```python
from build123d import *

# Parameters (mm, degrees)
BOSS_EXTRUDE1_DEPTH = 5
SKETCH1_13_R        = 1.1
CUT_EXTRUDE2_DEPTH  = 10
FILLET1_R           = 2
BOSS_EXTRUDE2_DEPTH = 14
SKETCH2_R           = 1.35
CUT_EXTRUDE3_DEPTH  = 110
FILLET2_R           = 5
CUT_EXTRUDE4_START  = 200
SKETCH2_3_R         = 2.75
CUT_EXTRUDE4_DEPTH  = 111


with BuildPart() as part:
    # Sketch1 → Boss-Extrude1 (new body)
    with BuildSketch(Plane.XY):
        with BuildLine():
            Line((27.361611466, 75.175409663), (32.833933759, 90.210491595))
            ThreePointArc((32.833933759, 90.210491595), (9.201192242, 95.558035043), (-15.017708644, 94.818080697))
            Line((-15.017708644, 94.818080697), (-12.514757203, 79.015067248))
            ThreePointArc((-12.514757203, 79.015067248), (7.667660202, 79.631695869), (27.361611466, 75.175409663))
        make_face()
    extrude(amount=BOSS_EXTRUDE1_DEPTH)

    # Sketch1<13> → Cut-Extrude2 (cut)
    with BuildSketch(Plane.XY):
        with BuildLine():
            ThreePointArc((13.453363993, 84.941197291), (19.959187303, 83.651843029), (26.346302102, 81.864964213))
            Line((26.346302102, 81.864964213), (27.571711502, 85.672636967))
            ThreePointArc((27.571711502, 85.672636967), (20.887521597, 87.542626426), (14.079101854, 88.891950654))
            Line((14.079101854, 88.891950654), (13.453363993, 84.941197291))
        make_face()
        with Locations((8, 88)):
            Circle(SKETCH1_13_R)
    extrude(amount=CUT_EXTRUDE2_DEPTH, mode=Mode.SUBTRACT)

    # Fillet1
    fillet1_edges = [part.edges().sort_by_distance(p)[0] for p in [
        (26.346302102, 81.864964213, 2.5),
        (27.571711502, 85.672636967, 2.5),
        (14.079101854, 88.891950654, 2.5),
        (13.453363993, 84.941197291, 2.5),
    ]]
    fillet(fillet1_edges, radius=FILLET1_R - 0.0001)  # a hair under: the kernel refuses the full size

    # Sketch1<14> → Boss-Extrude2 (add)
    with BuildSketch(Plane.XY):
        with BuildLine():
            ThreePointArc((-0.5, 93.344488005), (-9.226985142, 88), (-0.5, 82.655511995))
            Line((-0.5, 82.655511995), (-0.5, 93.344488005))
        make_face()
        with BuildLine():
            Line((-0.5, 93.344488005), (-0.5, 82.655511995))
            ThreePointArc((-0.5, 82.655511995), (1.889747744, 84.866464525), (2.773014858, 88))
            ThreePointArc((2.773014858, 88), (1.889747744, 91.133535475), (-0.5, 93.344488005))
        make_face()
    extrude(amount=BOSS_EXTRUDE2_DEPTH)

    # Sketch2 → Cut-Extrude3 (cut)
    with BuildSketch(Plane(origin=(0, 0, 0), x_dir=(1, 0, 0), z_dir=(0, 1, 0))):
        with Locations(Location((-3.226985142, -8, 0), (0, 0, 90))):
            Circle(SKETCH2_R)
    extrude(amount=CUT_EXTRUDE3_DEPTH, mode=Mode.SUBTRACT)

    # Fillet2
    fillet2_edges = [part.edges().sort_by_distance(p)[0] for p in [
        (27.361611466, 75.175409663, 2.5),
        (-12.514757203, 79.015067248, 2.5),
        (-15.017708644, 94.818080697, 2.5),
        (32.833933759, 90.210491595, 2.5),
    ]]
    fillet(fillet2_edges, radius=FILLET2_R)

    # Sketch2<3> → Cut-Extrude4 (cut)
    with BuildSketch(Plane(origin=(0, 0, 0), x_dir=(1, 0, 0), z_dir=(0, 1, 0)).offset(CUT_EXTRUDE4_START)):
        with Locations(Location((-3.226985142, -8, 0), (0, 0, 270))):
            Circle(SKETCH2_3_R)
    extrude(amount=-CUT_EXTRUDE4_DEPTH, mode=Mode.SUBTRACT)


solid = part.part
```
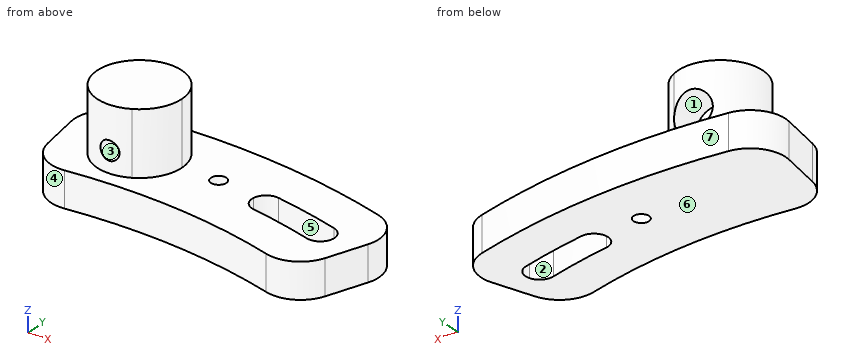
Work out the finished part from the listing and answer in its coordinate system (mm). Face numbers are marked on the shaded views. A direction names the side the tool comes from. Coordinates: 2 decimals unless noted, no trailing zeros. Order: outer loops, then holes, each group sorted by start corner. A loop starts at its lowest first (then second) coordinate and runs counter-clockwise, first axis right, second up. Notation, with made-up numbers: (79, 1.25) - (125, 1.25) arc R8 cw to (125, 6.25) - close; hole circle Ø3 at (-28, 40). An arc over 180 degrees is marked (long way). Answer as a JSON object with one key per item and string values.
1. Find section A-A on z = 1.5. Count the separate pieces of the cut face and the enclosed holes in it, plus the area to 3 significant figures.
Output values:
{"separate pieces": "1", "enclosed holes": "2", "area": "637 mm²"}
2. Find section C-C on y = 91. Determine the outline of the cut face in (x, z).
Output values:
{"outline": "(-14.25, 0) - (29.5, 0) - (29.5, 5) - (1.97, 5) - (1.97, 14) - (-8.42, 14) - (-8.42, 5) - (-14.25, 5) - close; hole circle Ø5.5 at (-3.23, 8)"}
3. Find section D-D on z = 11.25. Determine the outline of the cut face in (x, y).
Output values:
{"outline": "circle Ø12 at (-3.23, 88)"}
4. A tool of negligible diameter and unlimited length cuts with its end or side. For the marked faces 1, 2 and 3, from which of +Z, -Z, +X, -X, +Y, -Y can it reach the whole face along a straight path? Write none if from no direction.
Output values:
{"face 1": "+Y", "face 2": "+Z, -Z", "face 3": "+Y, -Y"}
5. Consider line 1 (Z direction, x = 15.5, y = 80.75); line 2 (X direction, y = 91.75, z = 8); line 3 (Y direction, x = 8, z = 3.3). Determine where each line is inside the solid, lowest interval first.
Output values:
{"line 1": "z = 0 to 5", "line 2": "x = -7.91 to -5.98, -0.48 to 1.46", "line 3": "y = 79.6 to 86.9, 89.1 to 95.67"}
6. Each of these flat-tipped pins is pushed along its axis until it touches: P1, Ø1, axis at x = 7.5, y = 80, coming from the +Z side; P2, Ø1, axis at y = 91.5, z = 6, coming from the -X side; P3, Ø8, axis at x = 23.5, z = 8, coming from the +Y side; P4, Ø10, axis at x = -7, y = 86, coming from the -Z side. Where does it stop, or does it pass through?
Output values:
{"P1": "stops at z = 5", "P2": "stops at x = -8.42", "P3": "stops at y = 93.71", "P4": "stops at z = 0"}
7. The mould has two halves that part along Y. Classify the marked faces 4, 5, 6 and 7: +Y half, -Y half, draft (parallel to the pull), parting line (faces both ways), or undercut.
Output values:
{"face 4": "-Y half", "face 5": "undercut", "face 6": "draft", "face 7": "+Y half"}
8. Find section B-B on x = 8. Determine the outline of the cut face in (y, z).
Output values:
{"outline": "(79.6, 0) - (86.9, 0) - (86.9, 5) - (79.6, 5) - close; (89.1, 0) - (95.67, 0) - (95.67, 5) - (89.1, 5) - close"}
